```python
from build123d import *

# Parameters (mm, degrees)
F0_W      = 34
F0_H      = 30
F1_DEPTH  = 20
F2_W      = 34
F2_H      = 24
F3_DEPTH  = 14
F5_D      = 4.2
F5_DEPTH  = 20
F5_TIP    = 1.2618073
F6_SIZE   = 5
F8_DEPTH  = 25
F9_D      = 6.6
F9_DEPTH  = 20
F9_TIP    = 1.9828400428
F10_W     = 34
F10_H     = 12
F11_DEPTH = 2.5


with BuildPart() as f1:
    # F0 (on Front) → F1 (new body)
    with BuildSketch(Plane.XZ):
        with Locations((17, 15)):
            Rectangle(F0_W, F0_H)
    extrude(amount=F1_DEPTH)

    # F2 (on face) → F3 (cut)
    with BuildSketch(Plane.XZ.offset(20)):
        with Locations((17, 12)):
            Rectangle(F2_W, F2_H)
    extrude(amount=-F3_DEPTH, mode=Mode.SUBTRACT)

    # F5
    with Locations(Plane(origin=(0, 0, 24), x_dir=(1, 0, 0), z_dir=(0, 0, -1))):
        with Locations((17, 15)):
            Hole(F5_D / 2, depth=F5_DEPTH)
            with Locations((0, 0, -(F5_DEPTH + F5_TIP / 2))):  # 118° drill point
                Cone(0, F5_D / 2, F5_TIP, mode=Mode.SUBTRACT)

    # F6
    f6_edges = [f1.edges().sort_by_distance(p)[0] for p in [
        (34, -20, 27),
        (0, -20, 27),
    ]]
    chamfer(f6_edges, length=F6_SIZE)

    # F7 (on face) → F8 (cut)
    with BuildSketch(Plane.XZ.offset(6)):
        with BuildLine():
            ThreePointArc((2.8578643763, 0), (14.4634703191, -19.7839783948), (32, -5))
            ThreePointArc((32, -5), (31.7839783948, -2.4634703191), (31.1421356237, 0))
            Line((31.1421356237, 0), (2.8578643763, 0))
        make_face()
        with BuildLine():
            Line((2.8578643763, 0), (31.1421356237, 0))
            ThreePointArc((31.1421356237, 0), (17, 10), (2.8578643763, 0))
        make_face()
    extrude(amount=-F8_DEPTH, mode=Mode.SUBTRACT)

    # F9
    with Locations(Plane.XZ.offset(6)):
        with Locations((5, 10), (29, 10)):
            Hole(F9_D / 2, depth=F9_DEPTH)
            with Locations((0, 0, -(F9_DEPTH + F9_TIP / 2))):  # 118° drill point
                Cone(0, F9_D / 2, F9_TIP, mode=Mode.SUBTRACT)

    # F10 (on face) → F11 (cut)
    with BuildSketch(Plane(origin=(0, 0, 0), x_dir=(-1, 0, 0), z_dir=(0, 1, 0))):
        with Locations((-17, 24)):
            Rectangle(F10_W, F10_H)
    extrude(amount=-F11_DEPTH, mode=Mode.SUBTRACT)


solid = f1.part
```
The model under review builds one solid part; all positions refer to its coordinate system, in mm. A direction names the side the tool comes from. Round coordinates to 2 decimals unless told otherwise and drop trailing zeros. Loops run counter-clockwise (first coordinate to the right, second up) from the corner with the lowest first, then second, coordinate; pieces in that order, holes last. Notation, with made-up numbers: M 1,-10 L 24,-10 A26 cw 24,25 Z; hole C 25.5,77.25 d9. An arc over 180 degrees is marked long. Put each result on its own line as item: value.
Q1. Mouldability with a two-part tool opening along Z and no side actions: class faces 4 (the flat face through (17, -12, 24)), 5 (the flat face through (17, -1, 18)), 6 (the cylindrical face through (3.48, -2.96, 7.07)), 7 (the flat face through (32, -17, 27)) as released by +Z, released by -Z, zero draft, split by the parting line, or undercut.
Result set:
face 4: released by -Z
face 5: released by +Z
face 6: undercut
face 7: zero draft
Q2. For pin 1 (4 mm diameter, centred on x = 5, z = 10, fed in from -Y); pin 2 (5.5 mm diameter, centred on x = 17, y = -15, fed in from -Z); pin 3 (2 mm diameter, centred on x = 9, y = -1, fed in from +Z); pin 4 (6 mm diameter, centred on x = 7, z = 20.5, fed in from -Y), all flat-tipped, find the tip position at first contact; note any pin that passes through.
Result set:
pin 1: passes through
pin 2: stops at z = 24
pin 3: stops at z = 18
pin 4: stops at y = -6
Q3. Consider section B-B, the plane z = 26.5. Give the boundary of the cut face in (x, y).
Result set:
outline: M 0,-15 L 5,-20 L 29,-20 L 34,-15 L 34,-2.5 L 0,-2.5 Z; hole C 17,-15 d4.2
Q4. Machinability: for faces 1 (the flat face through (17, -2.5, 24)), 2 (the flat face through (17, -20, 27)), 3 (the flat face through (17, -6, 15)), which of the approach directions +Z, -Z, +X, -X, +Y, -Y give a long, thin tool a straight path to every point of the face, cutting with its end or side? Answer none if there is none.
Result set:
face 1: +Z, +X, -X, +Y
face 2: +Z, -Z, +X, -X, -Y
face 3: -Z, +X, -X, -Y
Q5. Consider section C-C, the plane y = -5. Give the boundary of the cut face in (x, z), then the cut area to 3 significant figures.
Result set:
outline: M 0,0 L 2.86,0 A15 cw 31.14,0 L 34,0 L 34,30 L 0,30 Z; hole C 5,10 d6.6; hole C 29,10 d6.6
area: 745 mm²
Q6. To check wall thickness, follow L1, parallel to Y at x = 17, z = 26.6; L2, parallel to X at y = -15, z = 25.35; L3, parallel to Y at x = 21, z = 23.5. State the ranges of each line that lie inside material, in increasing order.
Result set:
L1: y = -20 to -17.1, -12.9 to -2.5
L2: x = 0 to 14.9, 19.1 to 34
L3: y = -6 to -2.5
Q7. Consider section D-D, the plane z = 7.5. Give the boundary of the cut face in (x, y), then the cut area to 3 significant figures.
Result set:
outline: M 0,-6 L 2.85,-6 L 2.85,0 L 0,0 Z; M 7.15,-6 L 8.71,-6 L 8.71,0 L 7.15,0 Z; M 25.29,-6 L 26.85,-6 L 26.85,0 L 25.29,0 Z; M 31.15,-6 L 34,-6 L 34,0 L 31.15,0 Z
area: 52.8 mm²
Q8. Consider section A-A, the plane x = 17. Give the boundary of the cut face in (y, z).
Result set:
outline: M -20,24 L -17.1,24 L -17.1,30 L -20,30 Z; M -12.9,24 L -6,24 L -6,10 L 0,10 L 0,18 L -2.5,18 L -2.5,30 L -12.9,30 Z
